from build123d import *

# Parameters (mm, degrees)
F0_R      = 7.5
F1_DEPTH  = 100
F2_R      = 3
F3_R      = 7.5
F3_R_2    = 4
F4_DEPTH  = 30
F5_R      = 3.5
F6_DEPTH  = 20
F1_FACE_R = 4
F7_DEPTH  = 23


with BuildPart() as f1:
    # F0 (on Top) → F1 (new body)
    with BuildSketch(Plane.XY):
        Circle(F0_R)
    extrude(amount=F1_DEPTH)

    # F2
    f2_edges = [f1.edges().sort_by_distance(p)[0] for p in [
        (-7.5, 0, 100),
    ]]
    fillet(f2_edges, radius=F2_R)

    # F3 (on face) → F4 (cut)
    with BuildSketch(Plane(origin=(0, 0, 0), x_dir=(1, 0, 0), z_dir=(0, 0, -1))):
        Circle(F3_R)
        Circle(F3_R_2, mode=Mode.SUBTRACT)
    extrude(amount=-F4_DEPTH, mode=Mode.SUBTRACT)

    # F5 (on Right) → F6 (join)
    with BuildSketch(Plane.YZ):
        with Locations((0, 36)):
            Circle(F5_R)
    extrude(amount=-F6_DEPTH)

    # F1_face (on face) → F7 (join)
    with BuildSketch(Plane(origin=(0, 0, 0), x_dir=(1, 0, 0), z_dir=(0, 0, -1))):
        Circle(F1_FACE_R)
    extrude(amount=F7_DEPTH)


solid = f1.part
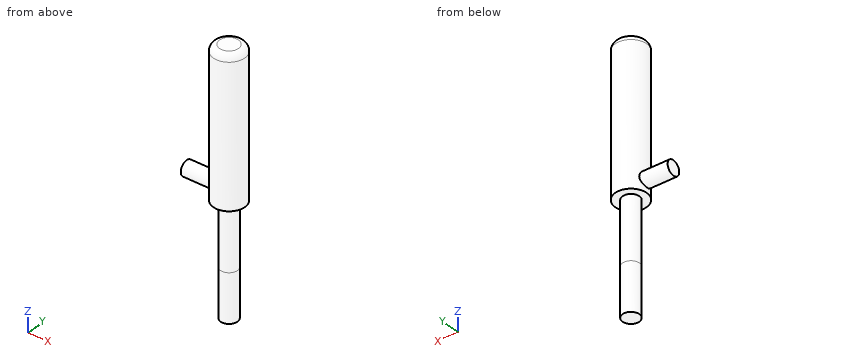
Build history of the part. All positions in model axes, mm. Round coordinates to 2 decimals unless told otherwise and drop trailing zeros. Loops run counter-clockwise (first coordinate to the right, second up) from the corner with the lowest first, then second, coordinate; pieces in that order, holes last. Notation, with made-up numbers: (-31.75, 32.25) -> (-12.75, 32.25) arc R24 ccw to (-12.75, 67.25) -> close; hole circle Ø8 at (59, 43.25). An arc over 180 degrees is marked (long way). Answer in a Markdown table with one row per item.
Item 1: Saw through at A-A (x = 0). Write the cut outline in (y, z), and give its area (3 significant figures).
Answers below:
| item | result |
|---|---|
| outline | (-7.5, 30) -> (-4, 30) -> (-4, -23) -> (4, -23) -> (4, 30) -> (7.5, 30) -> (7.5, 97) arc R3 ccw to (4.5, 100) -> (-4.5, 100) arc R3 ccw to (-7.5, 97) -> close |
| area | 1,470 mm² |
Item 2: Pin check, flat tips, straight feed: pin 1 (1.5 mm diameter, centred on y = -4, z = 11, fed in from -X); pin 2 (1.5 mm diameter, centred on x = -16.5, y = 2, fed in from +Z); pin 3 (5 mm diameter, centred on x = -12, y = 0.5, fed in from +Z). Stop position of each tip, or through.
Answers below:
| item | result |
|---|---|
| pin 1 | stops at x = -2.33 |
| pin 2 | stops at z = 39.27 |
| pin 3 | stops at z = 39.5 |
Item 3: Saw through at D-D (z = 72.5). Write the cut outline in (x, y), and give its area (3 significant figures).
Answers below:
| item | result |
|---|---|
| outline | circle Ø15 at (0, 0) |
| area | 177 mm² |
Item 4: Saw through at C-C (z = 36). Write the cut outline in (x, y), and give its area (3 significant figures).
Answers below:
| item | result |
|---|---|
| outline | (-20, -3.5) -> (-6.63, -3.5) arc R7.5 ccw (long way) to (-6.63, 3.5) -> (-20, 3.5) -> close |
| area | 266 mm² |
Item 5: Saw through at B-B (y = 0). Write the cut outline in (x, z), and give its area (3 significant figures).
Answers below:
| item | result |
|---|---|
| outline | (-20, 32.5) -> (-7.5, 32.5) -> (-7.5, 30) -> (-4, 30) -> (-4, -23) -> (4, -23) -> (4, 30) -> (7.5, 30) -> (7.5, 97) arc R3 ccw to (4.5, 100) -> (-4.5, 100) arc R3 ccw to (-7.5, 97) -> (-7.5, 39.5) -> (-20, 39.5) -> close |
| area | 1,560 mm² |
Item 6: Drill centre lines: L1, parallel to Z at x = -1, y = -4.75; L2, parallel to Y at x = -0.5, z = 93; L3, parallel to X at y = 0.25, z = 43. Where is each one in solid material? Low to high. Write a range as [from, to].
Answers below:
| item | result |
|---|---|
| L1 | z = [30, 99.98] |
| L2 | y = [-7.48, 7.48] |
| L3 | x = [-7.5, 7.5] |
